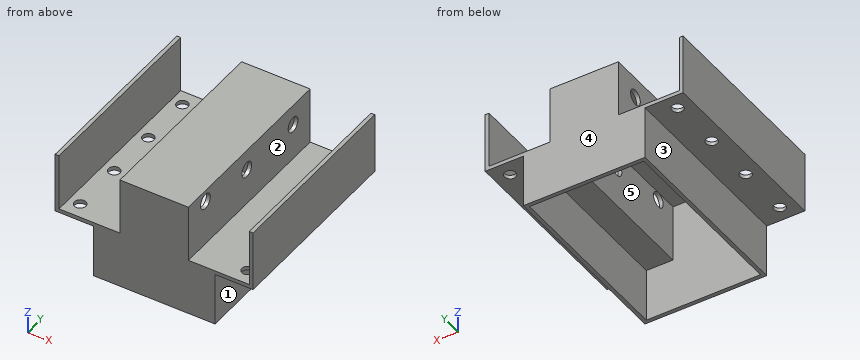
```python
from build123d import *

# Parameters (mm, degrees)
ESQUISSE1_W             = 90
ESQUISSE1_H             = 250
BOSS_EXTRU_1_DEPTH      = 5
ESQUISSE2_W             = 90
ESQUISSE2_H             = 250
ESQUISSE2_W_2           = 80
ESQUISSE2_H_2           = 240
BOSS_EXTRU_2_DEPTH      = 70
BOSS_EXTRU_3_DEPTH      = 5
ESQUISSE4_R             = 10
ENL_V_MAT_EXTRU_2_DEPTH = 171
ESQUISSE5_W             = 80
ESQUISSE5_H             = 250
BOSS_EXTRU_4_DEPTH      = 5
ESQUISSE6_W             = 80
ESQUISSE6_H             = 250
BOSS_EXTRU_5_DEPTH      = 5
ESQUISSE7_W             = 160
ESQUISSE7_H             = 250
ESQUISSE7_W_2           = 150
ESQUISSE7_H_2           = 240
BOSS_EXTRU_6_DEPTH      = 70
ESQUISSE10_R            = 7.5
ENL_V_MAT_EXTRU_3_DEPTH = 50


with BuildPart() as part:
    # Esquisse1 → Boss.-Extru.1 (new body)
    with BuildSketch(Plane.XY):
        with Locations((-45, 125)):
            Rectangle(ESQUISSE1_W, ESQUISSE1_H)
    extrude(amount=BOSS_EXTRU_1_DEPTH)

    # Esquisse2 → Boss.-Extru.2 (add)
    with BuildSketch(Plane(origin=(0, 0, 0), x_dir=(-1, 0, 0), z_dir=(0, 0, -1))):
        with Locations((45, 125)):
            Rectangle(ESQUISSE2_W, ESQUISSE2_H)
        with Locations((45, 125)):
            Rectangle(ESQUISSE2_W_2, ESQUISSE2_H_2, mode=Mode.SUBTRACT)
    extrude(amount=BOSS_EXTRU_2_DEPTH)

    # Esquisse3 → Boss.-Extru.3 (add)
    with BuildSketch(Plane(origin=(0, 0, -70), x_dir=(-1, 0, 0), z_dir=(0, 0, -1))):
        Polygon((6.025463364, 250), (-80, 250), (-80, 0), (-15, 0), (45, 0), (45, 5), (5, 5), (5, 245), (45, 245), (45, 250), align=None)
    boss_extru_3 = extrude(amount=BOSS_EXTRU_3_DEPTH)

    # Symétrie1: Boss.-Extru.3 across plane
    add(boss_extru_3.mirror(Plane(origin=(-45, 245, -75), x_dir=(0, 0, 1), z_dir=(1, 0, 0))))

    # Esquisse4 → Enlèv. mat.-Extru.2 (cut, through all)
    with BuildSketch(Plane.ZY.offset(90)):
        with Locations((-22, 215)):
            Circle(ESQUISSE4_R)
        with Locations((-22, 120)):
            Circle(ESQUISSE4_R)
        with Locations((-10, 35)):
            Circle(ESQUISSE4_R)
    extrude(amount=-ENL_V_MAT_EXTRU_2_DEPTH, mode=Mode.SUBTRACT)

    # Esquisse5 → Boss.-Extru.4 (add)
    with BuildSketch(Plane(origin=(80, 0, 0), x_dir=(0, 0, -1), z_dir=(1, 0, 0))):
        with Locations((35, 125)):
            Rectangle(ESQUISSE5_W, ESQUISSE5_H)
    extrude(amount=BOSS_EXTRU_4_DEPTH)

    # Esquisse6 → Boss.-Extru.5 (add)
    with BuildSketch(Plane.ZY.offset(170)):
        with Locations((-35, 125)):
            Rectangle(ESQUISSE6_W, ESQUISSE6_H)
    extrude(amount=BOSS_EXTRU_5_DEPTH)

    # Esquisse7 → Boss.-Extru.6 (add)
    with BuildSketch(Plane(origin=(0, 0, -75), x_dir=(-1, 0, 0), z_dir=(0, 0, -1))):
        with Locations((45, 125)):
            Rectangle(ESQUISSE7_W, ESQUISSE7_H)
        with Locations((45, 125)):
            Rectangle(ESQUISSE7_W_2, ESQUISSE7_H_2, mode=Mode.SUBTRACT)
    extrude(amount=BOSS_EXTRU_6_DEPTH)

    # Esquisse10 → Enlèv. mat.-Extru.3 (cut)
    with BuildSketch(Plane(origin=(0, 0, -75), x_dir=(-1, 0, 0), z_dir=(0, 0, -1))):
        with Locations((155, 230)):
            Circle(ESQUISSE10_R)
        with Locations((-65, 230)):
            Circle(ESQUISSE10_R)
        with Locations((-65, 160)):
            Circle(ESQUISSE10_R)
        with Locations((155, 160)):
            Circle(ESQUISSE10_R)
        with Locations((-65, 90)):
            Circle(ESQUISSE10_R)
        with Locations((155, 90)):
            Circle(ESQUISSE10_R)
        with Locations((-65, 20)):
            Circle(ESQUISSE10_R)
        with Locations((155, 20)):
            Circle(ESQUISSE10_R)
    extrude(amount=-ENL_V_MAT_EXTRU_3_DEPTH, mode=Mode.SUBTRACT)


solid = part.part
```
Could you check a few things on this model? Use its own coordinates, in mm. Face numbers are marked on the shaded views. A direction names the side the tool comes from. Give positions to 0.01 mm unless a question says otherwise; leave off trailing zeros. Loops run counter-clockwise (first coordinate to the right, second up) from the corner with the lowest first, then second, coordinate; pieces in that order, holes last. Notation, with made-up numbers: (61.5, 89.25) - (74.5, 89.25) arc R30 cw to (74.5, 125.25) - close; hole circle Ø10 at (39.5, 6). An arc over 180 degrees is marked (long way). Answer in a Markdown table with one row per item. Add a question column.
Q1. If we section it at D-D (z = -116): List the corners of the cut face in (x, y) for me, plus the area to 3 significant figures.
Q2. If we section it at A-A (z = -45.5): List the corners of the cut face in (x, y) for me, plus the area to 3 significant figures.
Q3. If we section it at C-C (x = 65): List the corners of the cut face in (y, z) for me.
Q4. Which directions (+Z, -Z, +X, -X, +Y, -Y) give clear straight access to the entire face, cutting with the end or side of a thin tool? Please do the marked faces 1, 2, 3, 4 and 5.
Q5. Please list where these lines run through material, in increasing order: L1, parallel to X at y = 222.5, z = -15; L2, parallel to Y at x = -155, z = -72.95; L3, parallel to Y at x = -2.55, z = -22. Write a range as from..to.
Q6. If we section it at B-B (y = 215): State how many separate pieces and enclosed holes the cut face has, plus the area to 3 significant figures.
Q7. For pin 1 (3 mm diameter, centred on x = -122.5, y = 162, fed in from +Z); pin 2 (3 mm diameter, centred on x = -146.5, y = 154, fed in from -Z); pin 3 (1 mm diameter, centred on y = 198.5, z = -109.5, fed in from +X), each with a flat end and sliding along its axis, tell me the tip position at first contact or that it passes through.
The answers:
| question | item | result |
|---|---|---|
| 1 | outline | (-125, 0) - (35, 0) - (35, 250) - (-125, 250) - close; hole (-120, 5) - (30, 5) - (30, 245) - (-120, 245) - close |
| 1 | area | 4,000 mm^2 |
| 2 | outline | (-175, 0) - (-170, 0) - (-170, 250) - (-175, 250) - close; (-90, 0) - (0, 0) - (0, 250) - (-90, 250) - close; (80, 0) - (85, 0) - (85, 250) - (80, 250) - close; hole (-85, 5) - (-5, 5) - (-5, 245) - (-85, 245) - close |
| 2 | area | 5,800 mm^2 |
| 3 | outline | (0, -75) - (12.5, -75) - (12.5, -70) - (0, -70) - close; (27.5, -75) - (82.5, -75) - (82.5, -70) - (27.5, -70) - close; (97.5, -75) - (152.5, -75) - (152.5, -70) - (97.5, -70) - close; (167.5, -75) - (222.5, -75) - (222.5, -70) - (167.5, -70) - close; (237.5, -75) - (250, -75) - (250, -70) - (237.5, -70) - close |
| 4 | face 1 | -Z, +X, +Y, -Y |
| 4 | face 2 | +Z, +Y, -Y |
| 4 | face 3 | -Z, -X, +Y, -Y |
| 4 | face 4 | +Z, -Z, +X, -X, +Y |
| 4 | face 5 | -Z |
| 5 | L1 | x = -175..-170, -90..-85, -5..0, 80..85 |
| 5 | L2 | y = 0..12.5, 27.5..82.5, 97.5..152.5, 167.5..222.5, 237.5..250 |
| 5 | L3 | y = 0..110, 130..205, 225..250 |
| 6 | separate pieces | 3 |
| 6 | enclosed holes | 0 |
| 6 | area | 3,300 mm^2 |
| 7 | pin 1 | stops at z = -70 |
| 7 | pin 2 | stops at z = -75 |
| 7 | pin 3 | stops at x = 35 |
